The figure shows three views and two pictorial views of one solid part (mm, origin at its lowest corner). Answer the questions. A direction names the side the tool comes from. Coordinates: 2 decimals unless noted, no trailing zeros. Order: outer loops, then holes, each group sorted by start corner. A loop starts at its lowest first (then second) coordinate and runs counter-clockwise, first axis right, second up.
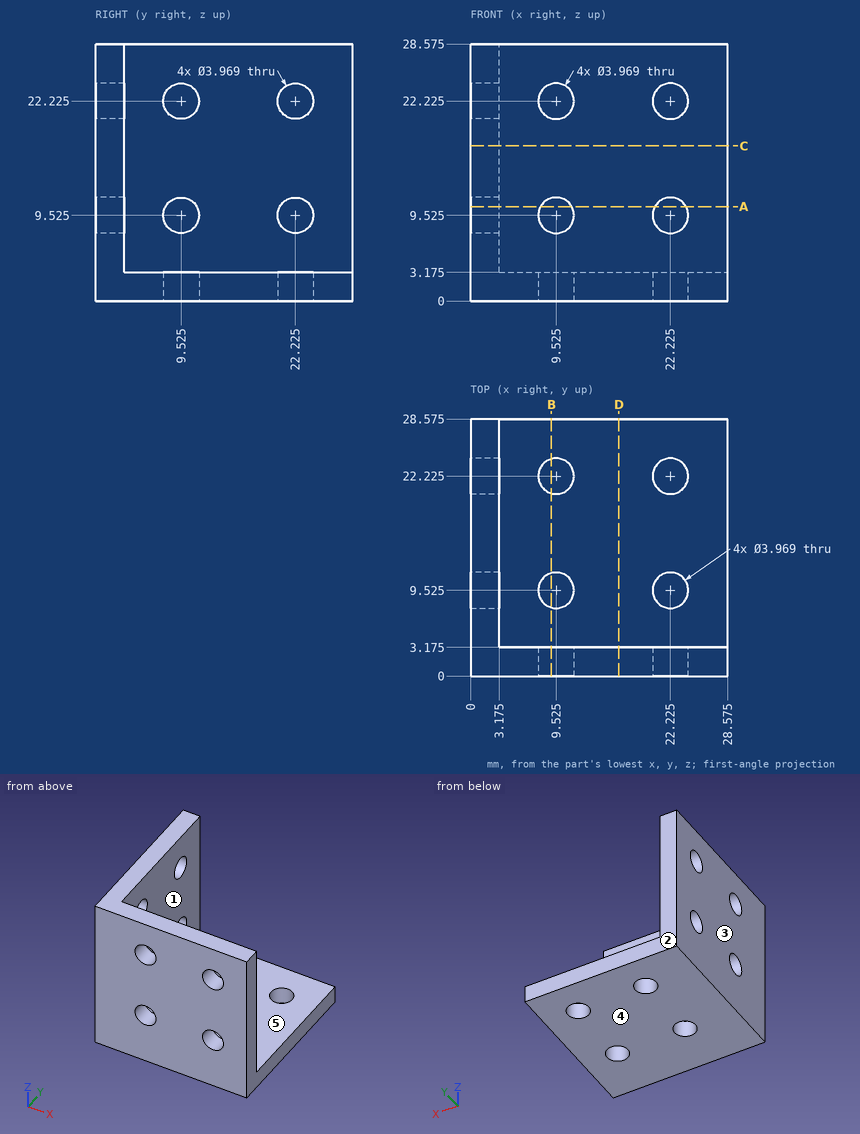
1) A cutting plane is placed at A-A, the plane z = 10.5. Write down the section's boundary in (x, y) (1 decimal).
2) A cutting plane is placed at B-B, the plane x = 9. Write down the section's boundary in (y, z) (1 decimal).
3) A straight line is drawn through the part: probe 1 along X at (y, z) = (6, 15) (1 decimal). Find the intervals that lie inside material, in ascending order.
4) For the marked faces 1 and 2, determine the directions among +Z, -Z, +X, -X, +Y, -Y from which every point of the face is accessible in a straight line to the end or side of a thin tool.
5) Each of these flat-tipped pins is pushed along its axis until it touches: P1, Ø12.5, axis at x = 14.5, z = 9.5, coming from the +Y side (3 decimals); P2, Ø5, axis at y = 9.525, z = 9.525, coming from the +X side (3 decimals); P3, Ø6.5, axis at x = 9.525, y = 22.225, coming from the +Z side (3 decimals). Where does it stop, or does it pass through?
6) A cutting plane is placed at C-C, the plane z = 17.25. Write down the section's boundary in (x, y) (1 decimal), plus the area to 3 significant figures.
7) The mould has two halves that part along Z. Classify the marked faces 3, 4 and 5: released by +Z, released by -Z, zero draft, split by the parting line, or undercut.
Working result:
1. outline: (0, 0) - (7.8, 0) - (7.8, 3.2) - (3.2, 3.2) - (3.2, 7.8) - (0, 7.8) - close; (0, 11.3) - (3.2, 11.3) - (3.2, 20.5) - (0, 20.5) - close; (0, 24) - (3.2, 24) - (3.2, 28.6) - (0, 28.6) - close; (11.3, 0) - (20.5, 0) - (20.5, 3.2) - (11.3, 3.2) - close; (24, 0) - (28.6, 0) - (28.6, 3.2) - (24, 3.2) - close
2. outline: (0, 0) - (7.6, 0) - (7.6, 3.2) - (3.2, 3.2) - (3.2, 7.6) - (0, 7.6) - close; (0, 11.4) - (3.2, 11.4) - (3.2, 20.3) - (0, 20.3) - close; (0, 24.1) - (3.2, 24.1) - (3.2, 28.6) - (0, 28.6) - close; (11.4, 0) - (20.3, 0) - (20.3, 3.2) - (11.4, 3.2) - close; (24.1, 0) - (28.6, 0) - (28.6, 3.2) - (24.1, 3.2) - close
3. probe 1: x = 0 to 3.2
4. face 1: +Z, +X, +Y
4. face 2: +Z, -Z, +X, -X, +Y
5. P1: stops at y = 3.175
5. P2: stops at x = 3.175
5. P3: stops at z = 3.175
6. outline: (0, 0) - (28.6, 0) - (28.6, 3.2) - (3.2, 3.2) - (3.2, 28.6) - (0, 28.6) - close
6. area: 171 mm2
7. face 3: zero draft
7. face 4: released by -Z
7. face 5: released by +Z
